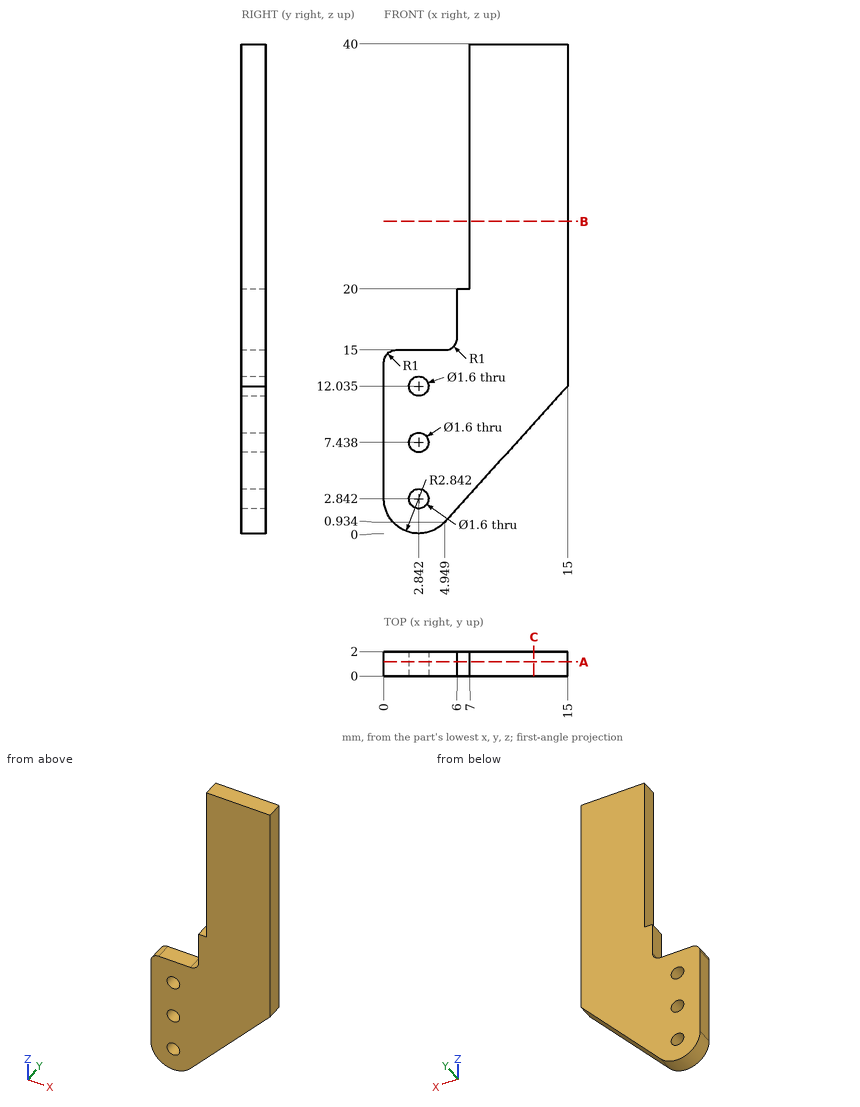
Verification items for this drawing (mm, ordinates from the low corner). Give positions to 0.01 mm unless a question says otherwise; leave off trailing zeros. Loops run counter-clockwise (first coordinate to the right, second up) from the corner with the lowest first, then second, coordinate; pieces in that order, holes last. Notation, with made-up numbers: M 24.25,-9 L 64.25,-9 A19 ccw 64.25,-4 Z; hole C 63.25,22.25 d8. An arc over 180 degrees is marked long. Answer in a Markdown table with one row per item.
1) Cross-section at B-B (z = 25.5). Enter the section's corners in (x, y).
Solutions:
| item | result |
|---|---|
| outline | M 7,0 L 15,0 L 15,2 L 7,2 Z |
2) Cross-section at A-A (y = 1.15). Enter the section's corners in (x, z) (1 decimal).
Solutions:
| item | result |
|---|---|
| outline | M 0,2.8 A2.8 ccw 4.9,0.9 L 15,12 L 15,40 L 7,40 L 7,20 L 6,20 L 6,16 A1 cw 5,15 L 1,15 A1 ccw 0,14 Z; hole C 2.8,2.8 d1.6; hole C 2.8,7.4 d1.6; hole C 2.8,12 d1.6 |
3) Thickness scan on line 1 (Z direction, x = 2.5, y = 1.8) (1 decimal); line 2 (Z direction, x = 3.5, y = 0.7) (1 decimal); line 3 (Z direction, x = 5, y = 0.15). Record the ranges inside material, lowest first.
Solutions:
| item | result |
|---|---|
| line 1 | z = 0 to 2.1, 3.6 to 6.7, 8.2 to 11.3, 12.8 to 15 |
| line 2 | z = 0.1 to 2.4, 3.3 to 7, 7.9 to 11.6, 12.5 to 15 |
| line 3 | z = 0.99 to 15 |
4) Depth check by flat-ended pin: pin 1 (0.5 mm diameter, centred on x = 6.5, y = 1, fed in from +Z); pin 2 (1 mm diameter, centred on y = 0.5, z = 32.5, fed in from -X); pin 3 (0.6 mm diameter, centred on y = 1.5, z = 17.5, fed in from -X). Enter the tip coordinate at first touch or a pass-through.
Solutions:
| item | result |
|---|---|
| pin 1 | stops at z = 20 |
| pin 2 | stops at x = 7 |
| pin 3 | stops at x = 6 |
5) Cross-section at C-C (x = 12.25). Enter the section's corners in (y, z).
Solutions:
| item | result |
|---|---|
| outline | M 0,9 L 2,9 L 2,40 L 0,40 Z |
